```python
from build123d import *

# Parameters (mm, degrees)
SKETCH_1_R               = 20
EXTRUDE_1_DEPTH          = 2
SKETCH_2_R               = 8
EXTRUDE_2_DEPTH          = 8.8
SKETCH_3_R               = 4
CUT_EXTRUDE_1_DEPTH      = 31.276063152
SKETCH_4_R               = 1.65
CUT_EXTRUDE_2_DEPTH      = 31.276063152
PATTERN_CIRCULAR_1_COUNT = 3


with BuildPart() as part:
    # 草图1 → 凸台-拉伸1 (new body)
    with BuildSketch(Plane.XY):
        Circle(SKETCH_1_R)
    extrude(amount=EXTRUDE_1_DEPTH)

    # 草图2 → 凸台-拉伸2 (add)
    with BuildSketch(Plane.XY.offset(2)):
        Circle(SKETCH_2_R)
    extrude(amount=EXTRUDE_2_DEPTH)

    # 草图3 → 切除-拉伸1 (cut, through all)
    with BuildSketch(Plane.XY.offset(10.8)):
        Circle(SKETCH_3_R)
    extrude(amount=-CUT_EXTRUDE_1_DEPTH, mode=Mode.SUBTRACT)

    # 草图4 → 切除-拉伸2 (cut, through all)
    with BuildSketch(Plane(origin=(0, 0, 0), x_dir=(-1, 0, 0), z_dir=(0, 0, -1))):
        with Locations((0, 15)):
            Circle(SKETCH_4_R)
    cut_extrude_2 = extrude(amount=-CUT_EXTRUDE_2_DEPTH, mode=Mode.SUBTRACT)

    # 阵列(圆周)1: 切除-拉伸2 ×3 about axis
    pattern_circular_1_axis = Axis((0, 0, 0), (0, 0, 1))
    for i in range(1, PATTERN_CIRCULAR_1_COUNT):
        add(cut_extrude_2.rotate(pattern_circular_1_axis, i * 360 / PATTERN_CIRCULAR_1_COUNT), mode=Mode.SUBTRACT)


solid = part.part
```
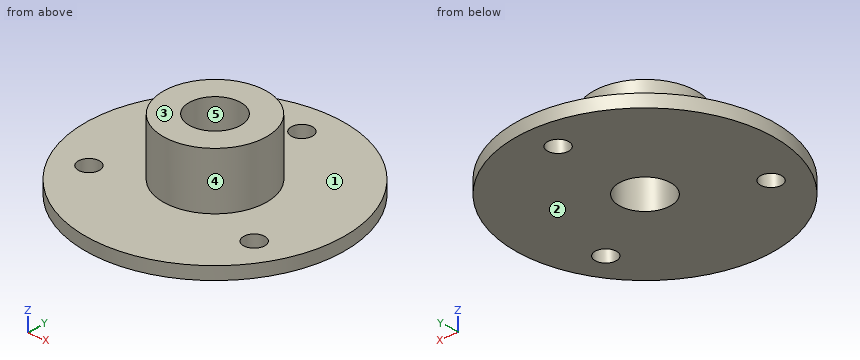
Check sheet for the modelled part. Datum: model origin and axes. Units: mm. Face numbers are marked on the shaded views. A direction names the side the tool comes from. Coordinates: 2 decimals unless noted, no trailing zeros. Write each loop counter-clockwise with the first axis right and the second up, starting at its lowest first coordinate (ties: lowest second). Pieces come first, ordered by that corner, then holes. Notation, with made-up numbers: M 0.5,16.5 L 55.5,16.5 A24 cw 55.5,52.5 Z; hole C 33,-7.5 d7. An arc over 180 degrees is marked long. Use one line per item in the form item = value.
Item 1: Sectioned sample at C-C, the plane x = 12.5. Record the cut outline in (y, z).
Answer below:
outline = M -15.61,0 L -9.08,0 L -9.08,2 L -15.61,2 Z; M -5.92,0 L 15.61,0 L 15.61,2 L -5.92,2 Z
Item 2: Release check for a two-part mould opening along X. For the marked faces 3, 4 and 5 record: pulls with the +X half, pulls with the -X half, needs draft (parallel to the pull), parting line crosses it, or undercut.
Answer below:
face_3 = needs draft
face_4 = parting line crosses it
face_5 = undercut
Item 3: Sectioned sample at D-D, the plane y = -7.5. Record the cut outline in (x, z).
Answer below:
outline = M -18.54,0 L -14.64,0 L -14.64,2 L -18.54,2 Z; M -11.34,0 L 11.34,0 L 11.34,2 L 2.78,2 L 2.78,10.8 L -2.78,10.8 L -2.78,2 L -11.34,2 Z; M 14.64,0 L 18.54,0 L 18.54,2 L 14.64,2 Z
Item 4: Set-up check for the marked faces 1 and 2: record each of +Z, -Z, +X, -X, +Y, -Y from which the full face is reachable in a straight line by a thin tool's end or side.
Answer below:
face_1 = +Z
face_2 = -Z, +X, -X, +Y, -Y
Item 5: Material ranges on L1, parallel to Y at x = 0, z = 1.45; L2, parallel to Y at x = 0, z = 4.5; L3, parallel to Z at x = 12.5, y = -5, recorded low to high. Write a range as from..to.
Answer below:
L1 = -20..-4, 4..13.35, 16.65..20
L2 = -8..-4, 4..8
L3 = 0..2
Item 6: Sectioned sample at B-B, the plane x = 0. Record the cut outline in (y, z), and give its area (3 significant figures).
Answer below:
outline = M -20,0 L -4,0 L -4,10.8 L -8,10.8 L -8,2 L -20,2 Z; M 4,0 L 13.35,0 L 13.35,2 L 8,2 L 8,10.8 L 4,10.8 Z; M 16.65,0 L 20,0 L 20,2 L 16.65,2 Z
area = 128 mm^2
Item 7: Sectioned sample at A-A, the plane y = 0. Record the cut outline in (x, z).
Answer below:
outline = M -20,0 L -4,0 L -4,10.8 L -8,10.8 L -8,2 L -20,2 Z; M 4,0 L 20,0 L 20,2 L 8,2 L 8,10.8 L 4,10.8 Z
Item 8: Gauge pin test, flat ends, axial feed: pin 1 Ø3 at (x, y) = (12.99, -7.5) entering from +Z; pin 2 Ø5 at (y, z) = (4, 3.5) entering from -X; pin 3 Ø4.5 at (x, y) = (-12.99, -7.5) entering from +Z; pin 4 Ø3 at (y, z) = (7.5, 9.5) entering from -X. Record the tip position at first contact, or that the pin passes through.
Answer below:
pin_1 = through
pin_2 = -19.9
pin_3 = 2
pin_4 = -5.29
